Answer from the drawing. Dimensions are ordinates in mm from the lowest x, y and z of the part. A direction names the side the tool comes from. Coordinates: 2 decimals unless noted, no trailing zeros. Write each loop counter-clockwise with the first axis right and the second up, starting at its lowest first coordinate (ties: lowest second). Pieces come first, ordered by that corner, then holes.
(1) For a pull along Z with two mould halves and no side action, classify the marked faces 4, 5 and 6 as +Z half, -Z half, draft (parallel to the pull), parting line (faces both ways), or undercut.
(2) Straight lines are drawn through the part: line 1 (Z direction, x = 50, y = 22.5); line 2 (X direction, y = 32.5, z = 34); line 3 (X direction, y = 32.5, z = 49.5). For each, find the intervals that lie inside material, in ascending order.
(3) Given P1, Ø5, axis at x = 13.5, y = 41, coming from the +Z side; P2, Ø8, axis at x = 21, y = 20.5, coming from the +Z side; P3, Ø12, axis at x = 80, z = 10.5, coming from the -Y side, each flat-ended and moving along its own axis, determine where each tip first touches the part or whether it passes through.
(4) The part is cut by section D-D on y = 22. Determine the outline of the cut face in (x, z).
(5) Which of the six approach directions +Z, -Z, +X, -X, +Y, -Y give full straight-line access (tool end or side, diameter ignored) to the marked faces 1, 2 and 3?
(6) The part is cut by section A-A on x = 50. Determine the outline of the cut face in (y, z).
(7) The part is cut by section C-C on y = 13. Determine the outline of the cut face in (x, z).
(8) The part is cut by section B-B on z = 50. Determine the outline of the cut face in (x, y), plus the area to 3 significant figures.
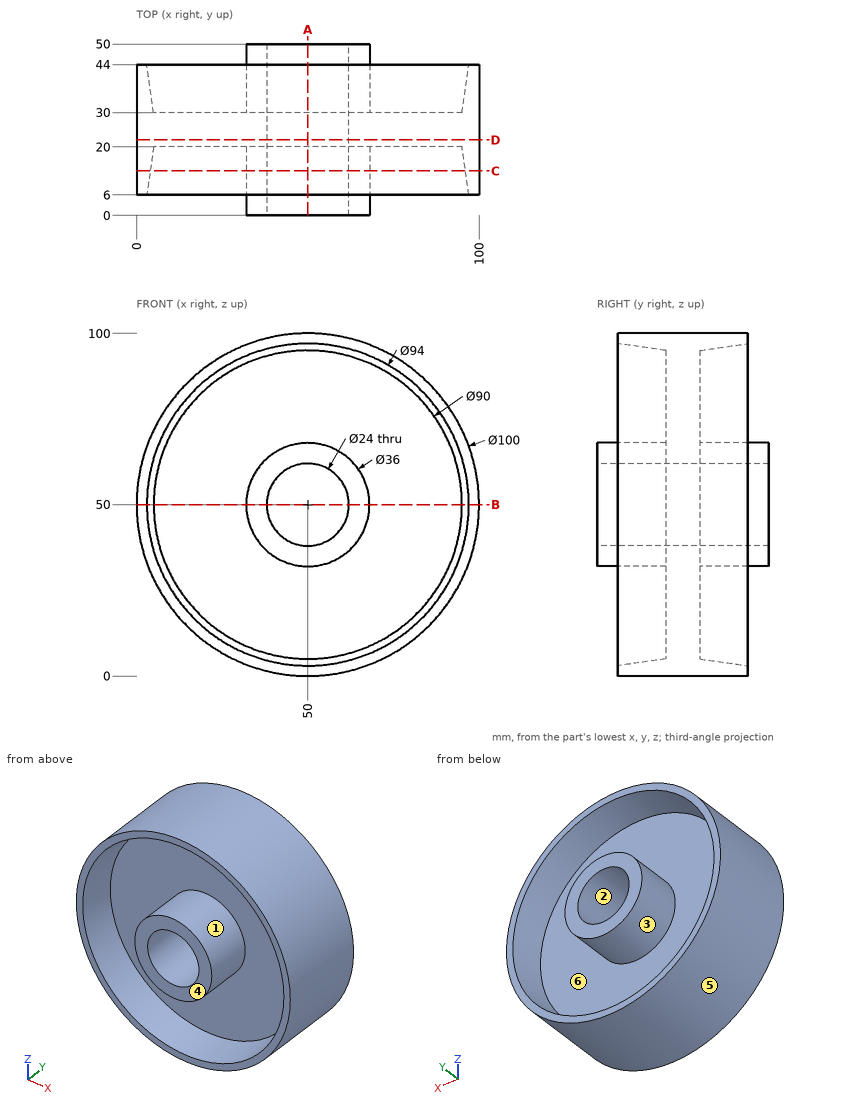
Model answer:
1. face 4: draft
1. face 5: parting line
1. face 6: undercut
2. line 1: z = 0 to 38, 62 to 100
2. line 2: x = 2.63 to 7.56, 41.75 to 58.25, 92.44 to 97.37
2. line 3: x = 0 to 4.65, 32.01 to 38.01, 61.99 to 67.99, 95.35 to 100
3. P1: stops at z = 86.66
3. P2: stops at z = 93.3
3. P3: stops at y = 6
4. outline: circle Ø100 at (50, 50); hole circle Ø24 at (50, 50)
5. face 1: -Y
5. face 2: +Y, -Y
5. face 3: +Y
6. outline: (0, 32) - (20, 32) - (20, 5) - (6, 3) - (6, 0) - (44, 0) - (44, 3) - (30, 5) - (30, 32) - (50, 32) - (50, 38) - (0, 38) - close; (0, 62) - (50, 62) - (50, 68) - (30, 68) - (30, 95) - (44, 97) - (44, 100) - (6, 100) - (6, 97) - (20, 95) - (20, 68) - (0, 68) - close
7. outline: circle Ø100 at (50, 50); circle Ø36 at (50, 50); hole circle Ø92 at (50, 50); hole circle Ø24 at (50, 50)
8. outline: (0, 6) - (3, 6) - (5, 20) - (32, 20) - (32, 0) - (38, 0) - (38, 50) - (32, 50) - (32, 30) - (5, 30) - (3, 44) - (0, 44) - close; (62, 0) - (68, 0) - (68, 20) - (95, 20) - (97, 6) - (100, 6) - (100, 44) - (97, 44) - (95, 30) - (68, 30) - (68, 50) - (62, 50) - close
8. area: 1,460 mm2
